Geometry: see drawing. Coordinates: mm, zero at the bounding-box minimum. Coordinates: 2 decimals unless noted, no trailing zeros. Write each loop counter-clockwise with the first axis right and the second up, starting at its lowest first coordinate (ties: lowest second). Pieces come first, ordered by that corner, then holes. Notation, with made-up numbers: (17.25, 9.5) - (73.25, 9.5) arc R20 ccw to (73.25, 25.5) - close; hole circle Ø11 at (37.5, 32). An arc over 180 degrees is marked (long way). One line per question, with ' | ' between items. Start each with the question number.
1) Section query C-C on y = 14. Return loops of the section in (x, z), and give its area (3 significant figures).
2) First-contact query: P1, Ø1.5, axis at y = 49, z = 1.5, coming from the -X side; P2, Ø4, axis at x = 19.5, y = 29.5, coming from the -Z side; P3, Ø1.5, axis at y = 2, z = 1, coming from the -X side; P4, Ø1.5, axis at x = 11.5, z = 1, coming from the +Y side. Flat tips, straight axial feed; report the tip coordinate or a pass-through.
3) Draft query along Z for the marked faces 1 and 2. Return one class per face: released by +Z, released by -Z, zero draft, split by the parting line, or undercut.
4) Line query: line 1 (X direction, y = 13, z = 2); line 2 (Y direction, x = 28, z = 1.45). Output: solid intervals per line, ascending.
5) Section query B-B on x = 15. Return loops of the section in (y, z), and give its area (3 significant figures).
6) Section query A-A on z = 0.7. Return loops of the section in (x, y).
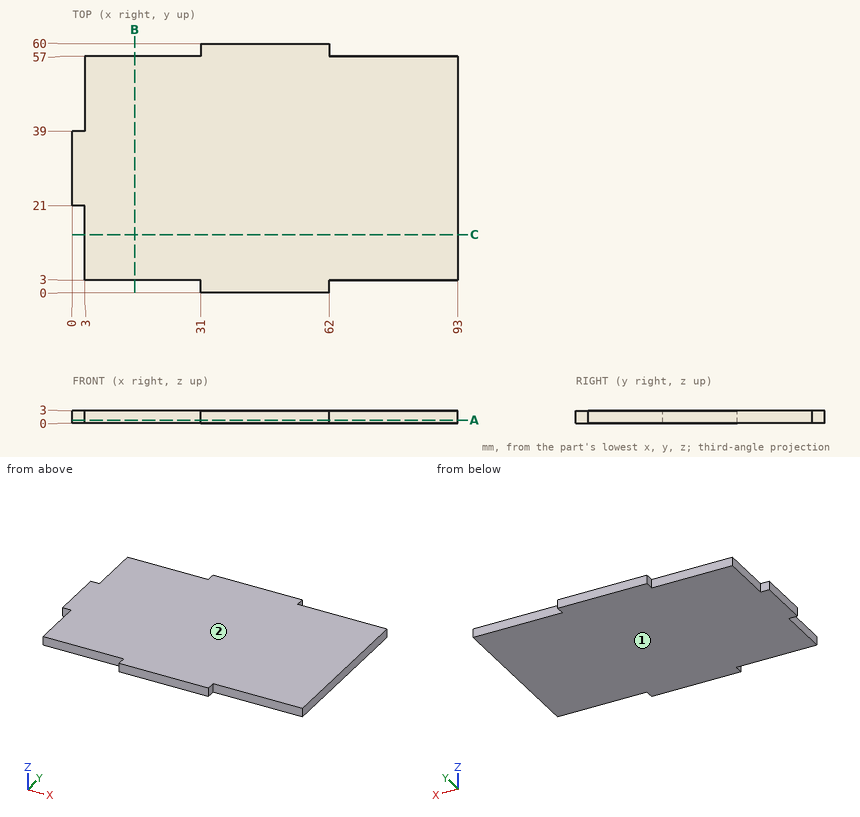
Answer key:
1) outline: (3, 0) - (93, 0) - (93, 3) - (3, 3) - close | area: 270 mm²
2) P1: x = 3 | P2: z = 0 | P3: x = 31 | P4: y = 57
3) face 1: released by -Z | face 2: released by +Z
4) line 1: 3 to 93 | line 2: 3 to 57
5) outline: (3, 0) - (57, 0) - (57, 3) - (3, 3) - close | area: 162 mm²
6) outline: (0, 21) - (3, 21) - (3, 3) - (31, 3) - (31, 0) - (62, 0) - (62, 3) - (93, 3) - (93, 57) - (62, 57) - (62, 60) - (31, 60) - (31, 57) - (3, 57) - (3, 39) - (0, 39) - close
